The model under review builds one solid part; all positions refer to its coordinate system, in mm. A direction names the side the tool comes from. Give positions to 0.01 mm unless a question says otherwise; leave off trailing zeros. Order: outer loops, then holes, each group sorted by start corner. A loop starts at its lowest first (then second) coordinate and runs counter-clockwise, first axis right, second up.
```python
from build123d import *

# Parameters (mm, degrees)
F0_W      = 50.8
F0_H      = 31.75
F1_DEPTH  = 31.75
F3_W      = 19.05
F3_H      = 19.05
F4_DEPTH  = 19.05
F5_W      = 19.0453663528
F5_H      = 19.05
F6_DEPTH  = 19.05
F8_DEPTH  = 25.4
F10_DEPTH = 25.4


with BuildPart() as f1:
    # F0 (on Front) → F1 (new body)
    with BuildSketch(Plane.XZ):
        with Locations((25.4, 15.875)):
            Rectangle(F0_W, F0_H)
    extrude(amount=F1_DEPTH)

    # F3 (on face) → F4 (cut)
    with BuildSketch(Plane.XZ.offset(31.75)):
        with Locations((9.525, 22.225)):
            Rectangle(F3_W, F3_H)
    extrude(amount=-F4_DEPTH, mode=Mode.SUBTRACT)

    # F5 (on face) → F6 (cut)
    with BuildSketch(Plane.XZ.offset(31.75)):
        with Locations((41.2773168236, 22.225)):
            Rectangle(F5_W, F5_H)
    extrude(amount=-F6_DEPTH, mode=Mode.SUBTRACT)

    # F7 (on face) → F8 (cut)
    with BuildSketch(Plane.YZ.offset(31.7546336472)):
        Polygon((-31.75, 31.75), (-31.75, 12.7), (-12.7, 31.75), align=None)
    extrude(amount=-F8_DEPTH, mode=Mode.SUBTRACT)

    # F9 (on face) → F10 (cut)
    with BuildSketch(Plane.XZ.offset(12.7)):
        Polygon((50.8, 31.75), (31.7546336472, 31.75), (50.8, 12.7), align=None)
    extrude(amount=-F10_DEPTH, mode=Mode.SUBTRACT)


solid = f1.part
```
Item 1: For line 1 (Y direction, x = 6.5, z = 25); line 2 (Z direction, x = 16, y = -14); line 3 (X direction, y = -21, z = 16), list the stretches that pass through material, from the lowest coordinate up.
Values found:
line 1: y = -12.7 to 0
line 2: z = 0 to 12.7
line 3: x = 19.05 to 31.75
Item 2: Take a section at D-D (x = 46.5). Give the boundary of the cut face in (y, z).
Values found:
outline: (-31.75, 0) - (0, 0) - (0, 17) - (-12.7, 17) - (-12.7, 12.7) - (-31.75, 12.7) - close
Item 3: Take a section at C-C (x = 15.5). Give the boundary of the cut face in (y, z).
Values found:
outline: (-31.75, 0) - (0, 0) - (0, 31.75) - (-12.7, 31.75) - (-12.7, 12.7) - (-31.75, 12.7) - close
Item 4: For faces 1 (the flat face through (19.05, -18, 18)), 2 (the flat face through (37, -12.7, 18)), 3 (the flat face through (41.1, -6.4, 22.4)), list the 3-axis set-ups (+Z, -Z, +X, -X, +Y, -Y) from which the entire face can be reached by the end or side of a thin tool; tool diameter is ignored.
Values found:
face 1: +Z, -X, -Y
face 2: +Z, +X, -Y
face 3: +Z, +X, +Y, -Y
Item 5: Take a section at A-A (y = -19). Give the boundary of the cut face in (x, z), and give its area (3 significant figures).
Values found:
outline: (0, 0) - (50.8, 0) - (50.8, 12.7) - (31.75, 12.7) - (31.75, 25.45) - (19.05, 25.45) - (19.05, 12.7) - (0, 12.7) - close
area: 807 mm2
Item 6: Take a section at B-B (z = 16). Give the boundary of the cut face in (x, y), and give its area (3 significant figures).
Values found:
outline: (0, -12.7) - (19.05, -12.7) - (19.05, -28.45) - (31.75, -28.45) - (31.75, -12.7) - (47.5, -12.7) - (47.5, 0) - (0, 0) - close
area: 803 mm2
Item 7: Clearance check with flat-ended pins moving along their axes: pin 1 Ø9.5 at (y, z) = (-20, 24) entering from +X; pin 2 Ø9.5 at (x, y) = (8, -26) entering from +Z; pin 3 Ø1 at (x, y) = (40, -13) entering from +Z. State where each tip first meets the part, or that it passes through.
Values found:
pin 1: stops at x = 31.75
pin 2: stops at z = 12.7
pin 3: stops at z = 23.9
